Work out the finished part from the listing and answer in its coordinate system (mm). Coordinates: 2 decimals unless noted, no trailing zeros. Write each loop counter-clockwise with the first axis right and the second up, starting at its lowest first coordinate (ties: lowest second). Pieces come first, ordered by that corner, then holes. Notation, with made-up numbers: (-17.75, 61.5) - (11.25, 61.5) arc R27 cw to (11.25, 97.5) - close; hole circle Ø5 at (35.25, -19.5). An arc over 180 degrees is marked (long way). Use one line per item in the form item = value. Start each with the question number.
Item 1: Given pin 1 (3 mm diameter, centred on x = -19.5, z = 2, fed in from +Y); pin 2 (1.5 mm diameter, centred on y = -1.5, z = 4.5, fed in from -X); pin 3 (1.5 mm diameter, centred on y = -18, z = 1.5, fed in from +X), each flat-ended and moving along its own axis, determine where each tip first touches the part or whether it passes through.
Item 2: Determine the mould class of faces 1 (the cylindrical face through (1.17, 35.54, 2.5)), 2 (the cylindrical face through (-9.845, -18.929, 2.504)), 3 (the flat face through (0, -24.892, 3)) for opening direction X: released by +X, released by -X, zero draft, split by the parting line, or undercut.
Item 3: A cutting plane is placed at A-A (y = 0). Write down the section's boundary in (x, z).
Item 4: A cutting plane is placed at B-B (x = 0). Write down the section's boundary in (y, z).
Item 5: Consider probe 1 along Y at (x, z) = (0, 2.4); probe 2 along Y at (x, z) = (-6.5, 0.9); probe 3 along X at (y, z) = (-9.5, 3.6). Determine where each line is inside the solid, lowest interval first.
Item 6: A cutting plane is placed at C-C (z = 1.3). Write down the section's boundary in (x, y).
from build123d import *

# Parameters (mm, degrees)
SKETCH1_R           = 35.56
BOSS_EXTRUDE1_DEPTH = 5.08
CUT_EXTRUDE1_DEPTH  = 51.545361805
SKETCH7_R           = 2.032
CUT_EXTRUDE2_DEPTH  = 51.545361805
SKETCH8_R           = 21.336
CUT_EXTRUDE3_DEPTH  = 51.545361805


with BuildPart() as part:
    # Sketch1 → Boss-Extrude1 (new body)
    with BuildSketch(Plane.XY):
        Circle(SKETCH1_R)
    extrude(amount=BOSS_EXTRUDE1_DEPTH)

    # Sketch2 → Cut-Extrude1 (cut, through all)
    with BuildSketch(Plane.XY.offset(5.08)):
        Polygon((0, -35.56), (-36.256055522, -35.56), (-36.256055522, -24.892), (33.75035888, -24.892), (33.75035888, -35.56), align=None)
    extrude(amount=-CUT_EXTRUDE1_DEPTH, mode=Mode.SUBTRACT)

    # Sketch7 → Cut-Extrude2 (cut, through all)
    with BuildSketch(Plane.XY.offset(5.08)):
        with Locations((-24.261099887, -20.626476503)):
            Circle(SKETCH7_R)
        with Locations((-7.471969114, 29.665523497)):
            Circle(SKETCH7_R)
        with Locations((25.522900113, -7.952823738)):
            Circle(SKETCH7_R)
    extrude(amount=-CUT_EXTRUDE2_DEPTH, mode=Mode.SUBTRACT)

    # Sketch8 → Cut-Extrude3 (cut, through all)
    with BuildSketch(Plane(origin=(0, 0, 0), x_dir=(-1, 0, 0), z_dir=(0, 0, -1))):
        Circle(SKETCH8_R)
    extrude(amount=-CUT_EXTRUDE3_DEPTH, mode=Mode.SUBTRACT)


solid = part.part
Answer:
q1.pin_1 = 30.67
q1.pin_2 = -35.55
q1.pin_3 = 31.1
q2.face_1 = split by the parting line
q2.face_2 = undercut
q2.face_3 = zero draft
q3.outline = (-35.56, 0) - (-21.34, 0) - (-21.34, 5.08) - (-35.56, 5.08) - close; (21.34, 0) - (35.56, 0) - (35.56, 5.08) - (21.34, 5.08) - close
q4.outline = (-24.89, 0) - (-21.34, 0) - (-21.34, 5.08) - (-24.89, 5.08) - close; (21.34, 0) - (35.56, 0) - (35.56, 5.08) - (21.34, 5.08) - close
q5.probe_1 = -24.89 to -21.34, 21.34 to 35.56
q5.probe_2 = -24.89 to -20.32, 20.32 to 27.88, 31.45 to 34.96
q5.probe_3 = -34.27 to -19.1, 19.1 to 24.21, 26.84 to 34.27
q6.outline = (-25.39, -24.89) - (25.39, -24.89) arc R35.56 ccw (long way) to start; hole circle Ø4.06 at (-24.26, -20.63); hole circle Ø42.67 at (0, 0); hole circle Ø4.06 at (-7.47, 29.67); hole circle Ø4.06 at (25.52, -7.95)
